Solid Edge part; units mm, degrees
sketch "Sketch1" plane through (0, 0, 0) normal (0, 0, 1) x (1, 0, 0)
  circle A0 centre (0, 0) radius 35.56
extrude "Protrusion1" add sketch "Sketch1" along normal blind 2.54
sketch "Sketch2" plane through (0, 0, 0) normal (0, 0, -1) x (1, 0, 0)
  line L0 (-33.1956, 12.75) -> (-23, 12.75)
  line L1 (-23, 12.75) -> (-23, 13.25)
  line L2 (-23, 13.25) -> (-24, 13.25)
  line L3 (-24, 13.25) -> (-24, 14.75)
  line L4 (-24, 14.75) -> (-23, 14.75)
  line L5 (-23, 14.75) -> (-23, 15.25)
  line L6 (-23, 15.25) -> (-32.124, 15.25)
  arc A0 (-32.124, 15.25) -> (-33.1956, 12.75) centre (0, 0) ccw
extrude "ExtrudedProtrusion_2" add sketch "Sketch2" against normal blind 20
extrude "Cutout1" [suppressed]
hole "Hole_5" at (0, 31, 2.54) direction (0, 0, -1) diameter 4.7625 end up to next
mirror "Mirror1" about plane through (0, 0, 0) normal (1, 0, 0) of "ExtrudedProtrusion_2"
pattern_circular "Pattern1" count 5 over 360 about axis through (0, 0, 2.54) along (0, 0, -1) of "Hole_5"
Source: CAD feature listing. Evaluate the final solid. Frame: model axes, mm. A direction names the side the tool comes from. Give positions to 0.01 mm unless a question says otherwise; leave off trailing zeros. Write each loop counter-clockwise with the first axis right and the second up, starting at its lowest first coordinate (ties: lowest second). Pieces come first, ordered by that corner, then holes. Notation, with made-up numbers: (56, 23.5) -> (81, 23.5) arc R23 ccw to (81, 40.5) -> close; hole circle Ø7 at (40, 78). An arc over 180 degrees is marked (long way). Return JSON: item names as keys, results as strings. Group by question number.
1. Section B-B, the plane z = 11.75. Output: boundary loops of the cut face in (x, y), then the cut area to 3 significant figures.
2. Section A-A, the plane x = 0. Output: boundary loops of the cut face in (y, z), then the cut area to 3 significant figures.
3. Access query for faces 4 (the face through (0.1, 33.38, 1.29)), 5 (the face through (28, -15.25, 11)). Directions: +Z, -Z, +X, -X, +Y, -Y. A direction counts if a zero-diameter tool reaches every point of the face in a straight line with its end or side. Return the directions, or none.
4. Pin query (flat end, axial travel): pin 1 Ø10 at (x, y) = (-22.5, -12) entering from -Z; pin 2 Ø5 at (y, z) = (-15.5, 12) entering from +X; pin 3 Ø6 at (x, z) = (-7, 4) entering from -Y; pin 4 Ø4 at (x, y) = (26, -22) entering from +Z. Return the tip coordinate at first contact, or that it passes through.
5. Section C-C, the plane y = 31. Output: boundary loops of the cut face in (x, z), then the cut area to 3 significant figures.
6. Material intervals for line 1 (Z direction, x = -18.5, y = 20); line 2 (X direction, y = -14, z = 17.25); line 3 (X direction, y = -1, z = 1.5), sorted ascending. Write a range as from..to.
7. Mould query, pull axis X, two halves, no side actions, for faces 1 (the face through (35.376, -3.61, 1.064)), 2 (the face through (0, 0, 0)), 3 (the face through (-31.73, 8.79, 1.29)). Classes: +X half, -X half, draft (parallel to the pull), parting line (faces both ways), or undercut.
Determined:
{
 "1": {"outline": "(-33.2, -12.75) arc R35.56 ccw to (-32.12, -15.25) -> (-23, -15.25) -> (-23, -14.75) -> (-24, -14.75) -> (-24, -13.25) -> (-23, -13.25) -> (-23, -12.75) -> close; (23, -15.25) -> (32.12, -15.25) arc R35.56 ccw to (33.2, -12.75) -> (23, -12.75) -> (23, -13.25) -> (24, -13.25) -> (24, -14.75) -> (23, -14.75) -> close", "area": "45.4 mm2"},
 "2": {"outline": "(-35.56, 0) -> (28.62, 0) -> (28.62, 2.54) -> (-35.56, 2.54) -> close; (33.38, 0) -> (35.56, 0) -> (35.56, 2.54) -> (33.38, 2.54) -> close", "area": "169 mm2"},
 "3": {"face 4": "+Z, -Z", "face 5": "+Z, +X, -X, -Y"},
 "4": {"pin 1": "stops at z = 0", "pin 2": "stops at x = 33.1", "pin 3": "stops at y = -35.29", "pin 4": "stops at z = 2.54"},
 "5": {"outline": "(-17.42, 0) -> (-2.38, 0) -> (-2.38, 2.54) -> (-17.42, 2.54) -> close; (2.38, 0) -> (17.42, 0) -> (17.42, 2.54) -> (2.38, 2.54) -> close", "area": "76.4 mm2"},
 "6": {"line 1": "z = 0..2.54", "line 2": "x = -32.69..-24, 24..32.69", "line 3": "x = -35.55..35.55"},
 "7": {"face 1": "parting line", "face 2": "draft", "face 3": "undercut"}
}
